Part model, mm, in its own coordinate system. A direction names the side the tool comes from. Give positions to 0.01 mm unless a question says otherwise; leave off trailing zeros. Write each loop counter-clockwise with the first axis right and the second up, starting at its lowest first coordinate (ties: lowest second). Pieces come first, ordered by that corner, then holes. Notation, with made-up numbers: M -26,47 L -21,47 A15 cw -21,74 Z; hole C -36.5,58 d10. An arc over 180 degrees is marked long. Use a Markdown table: item, result.
```python
from build123d import *

# Parameters (mm, degrees)
SKETCH1_R           = 2.15
SKETCH1_R_2         = 13.25
BOSS_EXTRUDE1_DEPTH = 2
SKETCH2_W           = 63.93
SKETCH2_H           = 60
SKETCH2_R           = 2
BOSS_EXTRUDE2_DEPTH = 2
BOSS_EXTRUDE3_DEPTH = 2
BOSS_EXTRUDE4_DEPTH = 2
FILLET1_R           = 2


with BuildPart() as part:
    # Sketch1 → Boss-Extrude1 (new body)
    with BuildSketch(Plane(origin=(0, 0, 0), x_dir=(0, 0, -1), z_dir=(1, 0, 0))):
        with BuildLine():
            Line((0, 0), (60, 0))
            Line((60, 0), (60, 30))
            ThreePointArc((60, 30), (30, 60), (0, 30))
            Line((0, 30), (0, 0))
        make_face()
        with Locations((30, 47.5)):
            Circle(SKETCH1_R, mode=Mode.SUBTRACT)
        with Locations((30, 30)):
            Circle(SKETCH1_R_2, mode=Mode.SUBTRACT)
        with Locations((47.5, 30)):
            Circle(SKETCH1_R, mode=Mode.SUBTRACT)
        with Locations((30, 12.5)):
            Circle(SKETCH1_R, mode=Mode.SUBTRACT)
        with Locations((12.5, 30)):
            Circle(SKETCH1_R, mode=Mode.SUBTRACT)
    extrude(amount=BOSS_EXTRUDE1_DEPTH)

    # Sketch2 → Boss-Extrude2 (add)
    with BuildSketch(Plane(origin=(0, 0, 0), x_dir=(1, 0, 0), z_dir=(0, 1, 0))):
        with Locations((-29.965, 30)):
            Rectangle(SKETCH2_W, SKETCH2_H)
        with Locations(Location((-12, 53, 0), (0, 0, 270))):
            Circle(SKETCH2_R, mode=Mode.SUBTRACT)
        with Locations(Location((-55.059526056, 53, 0), (0, 0, 270))):
            Circle(SKETCH2_R, mode=Mode.SUBTRACT)
        with Locations(Location((-55.059526056, 7, 0), (0, 0, 90))):
            Circle(SKETCH2_R, mode=Mode.SUBTRACT)
        with Locations(Location((-12, 7, 0), (0, 0, 90))):
            Circle(SKETCH2_R, mode=Mode.SUBTRACT)
        with BuildLine():
            Line((-21.85, 51), (-26.15, 51))
            ThreePointArc((-26.15, 51), (-28.15, 53), (-26.15, 55))
            Line((-26.15, 55), (-21.85, 55))
            ThreePointArc((-21.85, 55), (-19.85, 53), (-21.85, 51))
        make_face(mode=Mode.SUBTRACT)
        with BuildLine():
            Line((-41.15, 51), (-45.45, 51))
            ThreePointArc((-45.45, 51), (-47.45, 53), (-45.45, 55))
            Line((-45.45, 55), (-41.15, 55))
            ThreePointArc((-41.15, 55), (-39.15, 53), (-41.15, 51))
        make_face(mode=Mode.SUBTRACT)
        with BuildLine():
            Line((-41.15, 9), (-45.45, 9))
            ThreePointArc((-45.45, 9), (-47.45, 7), (-45.45, 5))
            Line((-45.45, 5), (-41.15, 5))
            ThreePointArc((-41.15, 5), (-39.15, 7), (-41.15, 9))
        make_face(mode=Mode.SUBTRACT)
        with BuildLine():
            Line((-21.85, 9), (-26.15, 9))
            ThreePointArc((-26.15, 9), (-28.15, 7), (-26.15, 5))
            Line((-26.15, 5), (-21.85, 5))
            ThreePointArc((-21.85, 5), (-19.85, 7), (-21.85, 9))
        make_face(mode=Mode.SUBTRACT)
        with BuildLine():
            Line((-22.15, 42.5), (-22.15, 17.5))
            ThreePointArc((-22.15, 17.5), (-24.15, 15.5), (-26.15, 17.5))
            Line((-26.15, 17.5), (-26.15, 42.5))
            ThreePointArc((-26.15, 42.5), (-24.15, 44.5), (-22.15, 42.5))
        make_face(mode=Mode.SUBTRACT)
        with BuildLine():
            Line((-41.45, 42.5), (-41.45, 17.5))
            ThreePointArc((-41.45, 17.5), (-43.45, 15.5), (-45.45, 17.5))
            Line((-45.45, 17.5), (-45.45, 42.5))
            ThreePointArc((-45.45, 42.5), (-43.45, 44.5), (-41.45, 42.5))
        make_face(mode=Mode.SUBTRACT)
    extrude(amount=BOSS_EXTRUDE2_DEPTH)

    # Sketch3 → Boss-Extrude3 (add)
    with BuildSketch(Plane(origin=(0, 0, -60), x_dir=(-1, 0, 0), z_dir=(0, 0, -1))):
        Polygon((0, 20.525104105), (23.871014094, 2), (0, 2), align=None)
    extrude(amount=-BOSS_EXTRUDE3_DEPTH)

    # Sketch4 → Boss-Extrude4 (add)
    with BuildSketch(Plane.XY):
        Polygon((0, 20.525104105), (-23.871014094, 2), (0, 2), align=None)
    extrude(amount=-BOSS_EXTRUDE4_DEPTH)

    # Fillet1
    fillet1_edges = [part.edges().sort_by_distance(p)[0] for p in [
        (-61.93, 1, 0),
        (-61.93, 1, -60),
        (2, 0, -30),
    ]]
    fillet(fillet1_edges, radius=FILLET1_R)


solid = part.part
```
1. Tool access for faces 4 (the flat face through (-13, 6, 0)), 5 (the cylindrical face through (-39.15, 0.99, -6.96)), 6 (the flat face through (-31, 2, -30)): list every direction of +Z, -Z, +X, -X, +Y, -Y with a clear straight run to the whole face (end or side of a thin tool).
Findings below:
| item | result |
|---|---|
| face 4 | +Z, +X, -X, +Y, -Y |
| face 5 | +Y, -Y |
| face 6 | -X, +Y |
2. Drill centre lines: L1, parallel to X at y = 10, z = -32; L2, parallel to Y at x = 0.55, z = -47.5. Where is each one in solid material? Low to high.
Findings below:
| item | result |
|---|---|
| L1 | 0 to 2 |
| L2 | 0.08 to 27.85, 32.15 to 54.37 |
3. Cut at D-D, the plane z = -12.5. Give the cut face in (x, y).
Findings below:
| item | result |
|---|---|
| outline | M -61.93,0 L 0,0 A2 ccw 2,2 L 2,27.85 L 0,27.85 L 0,2 L -61.93,2 Z; M 0,32.15 L 2,32.15 L 2,54.37 L 0,54.37 Z |
4. Cut at A-A, the plane x = -43.45. Give the cut face in (y, z), then the cut area to 3 significant figures.
Findings below:
| item | result |
|---|---|
| outline | M 0,-60 L 2,-60 L 2,-55 L 0,-55 Z; M 0,-51 L 2,-51 L 2,-44.5 L 0,-44.5 Z; M 0,-15.5 L 2,-15.5 L 2,-9 L 0,-9 Z; M 0,-5 L 2,-5 L 2,0 L 0,0 Z |
| area | 46.0 mm2 |
5. Cut at B-B, the plane z = -53. Give the cut face in (x, y), then the cut area to 3 significant figures.
Findings below:
| item | result |
|---|---|
| outline | M -61.93,0 L -57.06,0 L -57.06,2 L -61.93,2 Z; M -53.06,0 L -47.45,0 L -47.45,2 L -53.06,2 Z; M -39.15,0 L -28.15,0 L -28.15,2 L -39.15,2 Z; M -19.85,0 L -14,0 L -14,2 L -19.85,2 Z; M -10,0 L 0,0 A2 ccw 2,2 L 2,49.26 L 0,49.26 L 0,2 L -10,2 Z |
| area | 172 mm2 |
6. Cut at C-C, the plane y = 33. Give the cut face in (x, z), then the cut area to 3 significant figures.
Findings below:
| item | result |
|---|---|
| outline | M 0,-59.85 L 2,-59.85 L 2,-42.91 L 0,-42.91 Z; M 0,-17.09 L 2,-17.09 L 2,-0.15 L 0,-0.15 Z |
| area | 67.8 mm2 |
7. Two-plate mould, pull along Y, no slides. Class faces 1 (the cylindrical face through (0.99, 13.15, -32.05)), 2 (the cylindrical face through (-39.15, 0.99, -53.04)), 3 (the flat face through (-11.77, 11.39, -0.99)): released by +Y, released by -Y, zero draft, split by the parting line, or undercut.
Findings below:
| item | result |
|---|---|
| face 1 | undercut |
| face 2 | zero draft |
| face 3 | released by +Y |
8. Drop flat-ended pins along their axis: P1, Ø10, axis at y = 51, z = -18.5, coming from the -X side; P2, Ø2, axis at y = 28, z = -42, coming from the -X side; P3, Ø1.6, axis at y = 1, z = -29.5, coming from the +X side; P4, Ø1, axis at y = 0.5, z = -26.5, coming from the +X side. Give the stop position or say it passes through.
Findings below:
| item | result |
|---|---|
| P1 | x = 0 |
| P2 | through |
| P3 | x = 1.99 |
| P4 | x = 1.73 |
